Here's how the part is built. I have some questions about the finished solid (model axes, mm). Round coordinates to 2 decimals unless told otherwise and drop trailing zeros. Order: outer loops, then holes, each group sorted by start corner. A loop starts at its lowest first (then second) coordinate and runs counter-clockwise, first axis right, second up. Notation, with made-up numbers: M 86.25,18 L 128.25,18 A25 ccw 128.25,37 Z; hole C 47,-38 d3. An arc over 180 degrees is marked long. Write item = value, one per line. Start each with the question number.
Item 1: We'd pull the mould along X, two halves only. Please class faces 1 (the face through (-39.97, 3.04, 1.61)), 2 (the face through (1, 0, 22)), 3 (the face through (2.2, 3, -50.2)): pulls with the +X half, pulls with the -X half, needs draft (parallel to the pull), parting line crosses it, or undercut.
Item 2: Please list where these lines run through material, in increasing order: L1, parallel to X at y = 1.35, z = 0; L2, parallel to X at y = 3.65, z = 1; L3, parallel to X at y = 3.95, z = 8.
Item 3: I want a section at C-C, the plane x = 42.5. List the corners of the cut face in (y, z) for me.
Item 4: I want a section at A-A, the plane z = 0. List the corners of the cut face in (x, y) for me, plus the area to 3 significant figures.
Item 5: I'm going to push flat-ended pins straight in: P1, Ø6.5, axis at x = 26, z = 0, coming from the -Y side; P2, Ø3.5, axis at x = 42.5, z = 0, coming from the -Y side; P3, Ø1.5, axis at x = -35.5, y = 3, coming from the +Z side; P4, Ø1, axis at x = 35.5, y = 5, coming from the -Z side. Where does each tip first touch, or does it pass through?
Item 6: I want a section at D-D, the plane z = 26. List the corners of the cut face in (x, y) for me, plus the area to 3 significant figures.
Item 7: I want a section at B-B, the plane y = 2.7. State how many separate pieces and enclosed holes the cut face has, plus the area to 3 significant figures.
```python
from build123d import *

# Parameters (mm, degrees)
SKETCH_1_R          = 50.25
SKETCH_1_R_2        = 21
EXTRUDE_1_DEPTH     = 6
SKETCH_2_R          = 2.5
CUT_EXTRUDE_1_DEPTH = 6
SKETCH_3_R          = 3
CUT_EXTRUDE_2_DEPTH = 10
CHAMFER_1_SIZE      = 2


with BuildPart() as part:
    # Эскиз1 → Бобышка-Вытянуть1 (new body)
    with BuildSketch(Plane(origin=(0, 0, 0), x_dir=(1, 0, 0), z_dir=(0, 1, 0))):
        with Locations(Location((0, 0, 0), (0, 0, 270))):
            Circle(SKETCH_1_R)
        with Locations(Location((0, 0, 0), (0, 0, 270))):
            Circle(SKETCH_1_R_2, mode=Mode.SUBTRACT)
    extrude(amount=EXTRUDE_1_DEPTH)

    # Эскиз2 → Вырез-Вытянуть1 (cut)
    with BuildSketch(Plane(origin=(0, 6, 0), x_dir=(1, 0, 0), z_dir=(0, 1, 0))):
        with Locations(Location((0, 26, 0), (0, 0, 270))):
            Circle(SKETCH_2_R)
        with Locations(Location((-26, 0, 0), (0, 0, 270))):
            Circle(SKETCH_2_R)
        with Locations(Location((26, 0, 0), (0, 0, 270))):
            Circle(SKETCH_2_R)
        with Locations(Location((0, -26, 0), (0, 0, 270))):
            Circle(SKETCH_2_R)
    extrude(amount=-CUT_EXTRUDE_1_DEPTH, mode=Mode.SUBTRACT)

    # Эскиз3 → Вырез-Вытянуть2 (cut)
    with BuildSketch(Plane(origin=(0, 6, 0), x_dir=(1, 0, 0), z_dir=(0, 1, 0))):
        with Locations(Location((-42.5, 0, 0), (0, 0, 270))):
            Circle(SKETCH_3_R)
        with Locations(Location((0, 42.5, 0), (0, 0, 270))):
            Circle(SKETCH_3_R)
        with Locations(Location((42.5, 0, 0), (0, 0, 270))):
            Circle(SKETCH_3_R)
        with Locations(Location((0, -42.5, 0), (0, 0, 270))):
            Circle(SKETCH_3_R)
    extrude(amount=-CUT_EXTRUDE_2_DEPTH, mode=Mode.SUBTRACT)

    # Фаска1
    chamfer_1_edges = [part.edges().sort_by_distance(p)[0] for p in [
        (0, 6, -28.5),
        (-26, 6, -2.5),
        (26, 6, -2.5),
        (0, 6, 23.5),
    ]]
    chamfer(chamfer_1_edges, length=CHAMFER_1_SIZE)


solid = part.part
```
Filled in:
q1.face_1 = undercut
q1.face_2 = needs draft
q1.face_3 = parting line crosses it
q2.L1 = -50.25 to -45.5, -39.5 to -28.5, -23.5 to -21, 21 to 23.5, 28.5 to 39.5, 45.5 to 50.25
q2.L2 = -50.24 to -45.33, -39.67 to -28.29, -23.71 to -20.98, 20.98 to 23.71, 28.29 to 39.67, 45.33 to 50.24
q2.L3 = -49.61 to -19.42, 19.42 to 49.61
q3.outline = M 0,-26.81 L 6,-26.81 L 6,-3 L 0,-3 Z; M 0,3 L 6,3 L 6,26.81 L 0,26.81 Z
q4.outline = M -50.25,0 L -45.5,0 L -45.5,6 L -50.25,6 Z; M -39.5,0 L -28.5,0 L -28.5,4 L -30.5,6 L -39.5,6 Z; M -23.5,0 L -21,0 L -21,6 L -21.5,6 L -23.5,4 Z; M 21,0 L 23.5,0 L 23.5,4 L 21.5,6 L 21,6 Z; M 28.5,0 L 39.5,0 L 39.5,6 L 30.5,6 L 28.5,4 Z; M 45.5,0 L 50.25,0 L 50.25,6 L 45.5,6 Z
q4.area = 211 mm^2
q5.P1 = 0
q5.P2 = through
q5.P3 = 36.3
q5.P4 = -36.06
q6.outline = M -43,0 L -2.5,0 L -2.5,4 L -4.5,6 L -43,6 Z; M 2.5,0 L 43,0 L 43,6 L 4.5,6 L 2.5,4 Z
q6.area = 482 mm^2
q7.separate_pieces = 1
q7.enclosed_holes = 9
q7.area = 6,360 mm^2
